Verification items for the finished model (mm, model axes). Face numbers are marked on the shaded views. Round coordinates to 2 decimals unless told otherwise and drop trailing zeros. Loops run counter-clockwise (first coordinate to the right, second up) from the corner with the lowest first, then second, coordinate; pieces in that order, holes last. Notation, with made-up numbers: (67, 19.5) - (109, 19.5) arc R29 cw to (109, 50.5) - close; hole circle Ø11 at (76.5, 67.5). An arc over 180 degrees is marked (long way). Use CSV: the item, a comma, the result in double quotes.
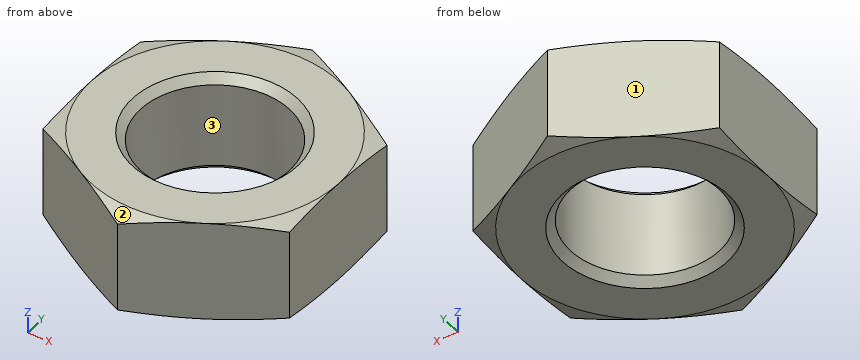
Autodesk Inventor part; units mm, degrees
ref_plane "NUT_XY" through (0, 0, 0) normal (0, 0, 1) x (1, 0, 0)
ref_plane "NUT_YZ" through (0, 0, 0) normal (1, 0, 0) x (0, 1, 0)
ref_plane "NUT_ZX" through (0, 0, 0) normal (0, 1, 0) x (0, 0, 1)
sketch "Sketch_8" plane through (0, 0, 0) normal (1, 0, 0) x (0, 1, 0)
  line L0 (0, -9.652) -> (0, 0)
  line L1 (0, 0) -> (11.938, 0)
  line L2 (11.938, 0) -> (14.3256, -0.6398)
  line L3 (14.3256, -0.6398) -> (14.3256, -9.0122)
  line L4 (14.3256, -9.0122) -> (11.938, -9.652)
  line L5 (11.938, -9.652) -> (0, -9.652)
  line L6 (0, -9.652) -> (0, 0)
sketch "Sketch_10" plane through (0, 0, 0) normal (0, 0, 1) x (1, 0, 0)
  line L0 (-23.876, -23.876) -> (23.876, -23.876)
  line L1 (23.876, -23.876) -> (23.876, 23.876)
  line L2 (23.876, 23.876) -> (-23.876, 23.876)
  line L3 (-23.876, 23.876) -> (-23.876, -23.876)
  line L4 (-11.938, -6.8924) -> (0, -13.7848)
  line L5 (0, -13.7848) -> (11.938, -6.8924)
  line L6 (11.938, -6.8924) -> (11.938, 6.8924)
  line L7 (11.938, 6.8924) -> (0, 13.7848)
  line L8 (0, 13.7848) -> (-11.938, 6.8924)
  line L9 (-11.938, 6.8924) -> (-11.938, -6.8924)
revolve "Revolution1" add sketch "Sketch_8" angle 360 about axis through (0, 0, -9.652) along (0, 0, -1)
extrude "Extrusion1" cut sketch "Sketch_10" against normal blind 9.652
sketch "Sketch_11" plane through (0, 0, 0) normal (1, 0, 0) x (0, 1, 0)
  line L0 (0, -9.652) -> (0, 0)
  line L1 (0, 0) -> (7.9375, 0)
  line L2 (7.9375, 0) -> (7.1742, -0.7633)
  line L3 (7.1742, -0.7633) -> (7.1742, -8.8887)
  line L4 (7.1742, -8.8887) -> (7.9375, -9.652)
  line L5 (7.9375, -9.652) -> (0, -9.652)
  line L6 (0, -9.652) -> (0, 0)
revolve "Revolution2" cut sketch "Sketch_11" angle 360 about axis through (0, 0, -9.652) along (0, 0, -1)
thread "Thread1"
ref_plane "NUT_XY" through (0, 0, 0) normal (0, 0, 1) x (1, 0, 0)
ref_plane "NUT_YZ" through (0, 0, 0) normal (1, 0, 0) x (0, 1, 0)
ref_plane "NUT_ZX" through (0, 0, 0) normal (0, 1, 0) x (0, 0, 1)
ref_plane "a1_XY" through (-11.938, 11.938, 0) normal (0, 0, 1) x (1, 0, 0)
ref_plane "a1_YZ" through (-11.938, 11.938, 0) normal (1, 0, 0) x (0, 1, 0)
ref_plane "a1_ZX" through (-11.938, 11.938, 0) normal (0, 1, 0) x (0, 0, 1)
ref_plane "a2_XY" through (11.938, 11.938, 0) normal (0, 0, 1) x (1, 0, 0)
ref_plane "a2_YZ" through (11.938, 11.938, 0) normal (1, 0, 0) x (0, 1, 0)
ref_plane "a2_ZX" through (11.938, 11.938, 0) normal (0, 1, 0) x (0, 0, 1)
ref_plane "b1_XY" through (0, 11.938, 0) normal (1, 0, 0) x (0, 0, -1)
ref_plane "b1_YZ" through (0, 11.938, 0) normal (0, 0, -1) x (0, 1, 0)
ref_plane "b1_ZX" through (0, 11.938, 0) normal (0, 1, 0) x (1, 0, 0)
ref_plane "b2_XY" through (0, 11.938, -9.652) normal (1, 0, 0) x (0, 0, -1)
ref_plane "b2_YZ" through (0, 11.938, -9.652) normal (0, 0, -1) x (0, 1, 0)
ref_plane "b2_ZX" through (0, 11.938, -9.652) normal (0, 1, 0) x (1, 0, 0)
ref_plane "e_XY" through (0, 0, -9.652) normal (1, 0, 0) x (0, 0, -1)
ref_plane "e_YZ" through (0, 0, -9.652) normal (0, 0, -1) x (0, 1, 0)
ref_plane "e_ZX" through (0, 0, -9.652) normal (0, 1, 0) x (1, 0, 0)
ref_plane "ol1_XY" through (0, 0, -11.938) normal (0, 1, 0) x (1, 0, 0)
ref_plane "ol1_YZ" through (0, 0, -11.938) normal (1, 0, 0) x (0, 0, -1)
ref_plane "ol1_ZX" through (0, 0, -11.938) normal (0, 0, -1) x (0, 1, 0)
ref_plane "ol2_XY" through (9.652, 0, -11.938) normal (0, 1, 0) x (1, 0, 0)
ref_plane "ol2_YZ" through (9.652, 0, -11.938) normal (1, 0, 0) x (0, 0, -1)
ref_plane "ol2_ZX" through (9.652, 0, -11.938) normal (0, 0, -1) x (0, 1, 0)
ref_plane "th1_XY" through (0, 7.9375, -9.652) normal (1, 0, 0) x (0, 0, -1)
ref_plane "th1_YZ" through (0, 7.9375, -9.652) normal (0, 0, -1) x (0, 1, 0)
ref_plane "th1_ZX" through (0, 7.9375, -9.652) normal (0, 1, 0) x (1, 0, 0)
ref_plane "th2_XY" through (0, -7.9375, -9.652) normal (1, 0, 0) x (0, 0, -1)
ref_plane "th2_YZ" through (0, -7.9375, -9.652) normal (0, 0, -1) x (0, 1, 0)
ref_plane "th2_ZX" through (0, -7.9375, -9.652) normal (0, 1, 0) x (1, 0, 0)
properties part number "D-9" material "Steel, Galvanized"
1) Cross-section at A-A, the plane z = -4. Record the cut outline in (x, y), then the cut area to 3 significant figures.
Returned:
outline,"(-11.94, -6.89) - (0, -13.78) - (11.94, -6.89) - (11.94, 6.89) - (0, 13.78) - (-11.94, 6.89) - close; hole circle Ø14.35 at (0, 0)"
area,"332 mm²"
2) Thickness scan on probe 1 along X at (y, z) = (0, -4.5); probe 2 along X at (y, z) = (6, -9); probe 3 along Y at (x, z) = (3, -5.75). Record the ranges inside material, lowest first. Write a range as [from, to].
Returned:
probe 1,"x = [-11.94, -7.17], [7.17, 11.94]"
probe 2,"x = [-11.94, -4.13], [4.13, 11.94]"
probe 3,"y = [-12.05, -6.52], [6.52, 12.05]"
3) Mould release check, pull along X, two halves, no side actions. Record for the marked faces 1, 2 and 3: +X half, -X half, draft (parallel to the pull), parting line (faces both ways), or undercut.
Returned:
face 1,"-X half"
face 2,"parting line"
face 3,"undercut"
4) Gauge pin test, flat ends, axial feed: pin 1 Ø3 at (x, z) = (-4.5, -2) entering from +Y; pin 2 Ø4 at (x, z) = (-0.5, -6) entering from -Y. Record the tip position at first contact, or that the pin passes through.
Returned:
pin 1,"stops at y = 12.05"
pin 2,"stops at y = -13.78"
